from build123d import *

# Parameters (mm, degrees)
F0_R     = 13
F0_R_2   = 7
F1_DEPTH = 4
F2_R     = 0.75
F3_DEPTH = 2
F4_R     = 0.5
F5_R     = 10.5
F5_R_2   = 9
F6_DEPTH = 2


with BuildPart() as f1:
    # F0 (on Top) → F1 (new body)
    with BuildSketch(Plane.XY):
        Circle(F0_R)
        Circle(F0_R_2, mode=Mode.SUBTRACT)
    extrude(amount=F1_DEPTH)

    # F2 (on Top) → F3 (join)
    with BuildSketch(Plane.XY):
        with Locations((0, -10)):
            Circle(F2_R)
        with Locations((-10, 0)):
            Circle(F2_R)
        with Locations((0, 10)):
            Circle(F2_R)
        with Locations((10, 0)):
            Circle(F2_R)
    extrude(amount=-F3_DEPTH)

    # F4
    f4_edges = [f1.edges().sort_by_distance(p)[0] for p in [
        (-10.75, 0, -2),
        (-0.75, -10, -2),
        (9.25, 0, -2),
        (-0.75, 10, -2),
    ]]
    fillet(f4_edges, radius=F4_R)

    # F5 (on face) → F6 (cut)
    with BuildSketch(Plane.XY.offset(4)):
        Circle(F5_R)
        Circle(F5_R_2, mode=Mode.SUBTRACT)
    extrude(amount=-F6_DEPTH, mode=Mode.SUBTRACT)


solid = f1.part
Geometry check sheet. Reference: the model listing, model coordinates, mm. A direction names the side the tool comes from. Coordinates: 2 decimals unless noted, no trailing zeros. Write each loop counter-clockwise with the first axis right and the second up, starting at its lowest first coordinate (ties: lowest second). Pieces come first, ordered by that corner, then holes. Notation, with made-up numbers: (18.5, 40.25) -> (34.5, 40.25) arc R12 cw to (34.5, 53.25) -> close; hole circle Ø7 at (-5, 39). An arc over 180 degrees is marked (long way). One line per question, with ' | ' between items.
1. Cross-section at A-A on y = -1.5. Record the cut outline in (x, z).
Answers:
outline: (-12.91, 0) -> (-6.84, 0) -> (-6.84, 4) -> (-8.87, 4) -> (-8.87, 2) -> (-10.39, 2) -> (-10.39, 4) -> (-12.91, 4) -> close; (6.84, 0) -> (12.91, 0) -> (12.91, 4) -> (10.39, 4) -> (10.39, 2) -> (8.87, 2) -> (8.87, 4) -> (6.84, 4) -> close
2. Cross-section at C-C on x = 3.25. Record the cut outline in (y, z), and give its area (3 significant figures).
Answers:
outline: (-12.59, 0) -> (-6.2, 0) -> (-6.2, 4) -> (-8.39, 4) -> (-8.39, 2) -> (-9.98, 2) -> (-9.98, 4) -> (-12.59, 4) -> close; (6.2, 0) -> (12.59, 0) -> (12.59, 4) -> (9.98, 4) -> (9.98, 2) -> (8.39, 2) -> (8.39, 4) -> (6.2, 4) -> close | area: 44.7 mm²
3. Depth check by flat-ended pin: pin 1 Ø3 at (x, z) = (-5, 1.5) entering from -Y; pin 2 Ø12.5 at (x, y) = (0, 0) entering from -Z; pin 3 Ø3 at (y, z) = (-7.5, 0) entering from -X; pin 4 Ø2 at (x, z) = (-3, 2.5) entering from +Y. Enter the tip coordinate at first touch or a pass-through.
Answers:
pin 1: stops at y = -12.52 | pin 2: passes through | pin 3: stops at x = -11.53 | pin 4: stops at y = 12.85
4. Set-up check for faces 4 (the cylindrical face through (-0.098, -9.256, -0.74)), 5 (the cylindrical face through (-10.316, -7.91, 1.972)), 6 (the cylindrical face through (-1.172, 8.923, 3.014)): record each of +Z, -Z, +X, -X, +Y, -Y from which the full face is reachable in a straight line by a thin tool's end or side.
Answers:
face 4: -Z | face 5: +Z, -Z | face 6: +Z
5. Thickness scan on probe 1 along Y at (x, z) = (0, 3.1); probe 2 along X at (y, z) = (5.75, 2.2); probe 3 along Y at (x, z) = (0, 1.95). Record the ranges inside material, lowest first. Write a range as from..to.
Answers:
probe 1: y = -13..-10.5, -9..-7, 7..9, 10.5..13 | probe 2: x = -11.66..-8.79, -6.92..-3.99, 3.99..6.92, 8.79..11.66 | probe 3: y = -13..-7, 7..13
6. Draft check along Y on faces 1 (the cylindrical face through (9.25, 0.03, -0.74)), 2 (the flat face through (-9, 6, 4)), 3 (the flat face through (8, 5, 2)). Enter one of: +Y half, -Y half, draft (parallel to the pull), parting line (faces both ways), or undercut.
Answers:
face 1: parting line | face 2: draft | face 3: undercut
7. Cross-section at D-D on x = -7.75. Record the cut outline in (y, z), and give its area (3 significant figures).
Answers:
outline: (-10.44, 0) -> (10.44, 0) -> (10.44, 4) -> (7.08, 4) -> (7.08, 2) -> (4.58, 2) -> (4.58, 4) -> (-4.58, 4) -> (-4.58, 2) -> (-7.08, 2) -> (-7.08, 4) -> (-10.44, 4) -> close | area: 73.5 mm²
8. Cross-section at B-B on z = 3.05. Record the cut outline in (x, y).
Answers:
outline: circle Ø26 at (0, 0); circle Ø18 at (0, 0); hole circle Ø21 at (0, 0); hole circle Ø14 at (0, 0)
